Design review of the part built by this model. Coordinates are the model's own, in mm. Round coordinates to 2 decimals unless told otherwise and drop trailing zeros. Loops run counter-clockwise (first coordinate to the right, second up) from the corner with the lowest first, then second, coordinate; pieces in that order, holes last. Notation, with made-up numbers: (-27, -22) -> (21, -22) arc R30 ccw to (21, 16) -> close; hole circle Ø1 at (10.25, -25). An arc over 180 degrees is marked (long way). Answer as CSV lines item,"result". Start each with the question number.
```python
from build123d import *

# Parameters (mm, degrees)
BOSS_EXTRUDE1_DEPTH = 4
SKETCH2_W           = 165.1
SKETCH2_H           = 63.5
CUT_EXTRUDE1_DEPTH  = 349.523826216
CUT_EXTRUDE2_DEPTH  = 10


with BuildPart() as part:
    # Sketch1 → Boss-Extrude1 (new body)
    with BuildSketch(Plane(origin=(0, 0, 0), x_dir=(1, 0, 0), z_dir=(0, 1, 0))):
        Polygon((310, -100), (310, -10), (280.7, -10), (280.7, -6), (310, -6), (310, 0), (0, 0), (0, -6), (29.3, -6), (29.3, -10), (0, -10), (0, -100), (153, -159.225806452), (153, -128.4), (157, -128.4), (157, -159.225806452), align=None)
    extrude(amount=BOSS_EXTRUDE1_DEPTH)

    # Sketch2 → Cut-Extrude1 (cut, through all)
    with BuildSketch(Plane(origin=(0, 4, 0), x_dir=(1, 0, 0), z_dir=(0, 1, 0))):
        with Locations((155, -31.75)):
            Rectangle(SKETCH2_W, SKETCH2_H)
    extrude(amount=-CUT_EXTRUDE1_DEPTH, mode=Mode.SUBTRACT)

    # Sketch4 → Cut-Extrude2 (cut)
    with BuildSketch(Plane(origin=(0, 4, 0), x_dir=(1, 0, 0), z_dir=(0, 1, 0))):
        with BuildLine():
            ThreePointArc((73.3, -97.8), (73.429171307, -98.929171307), (73.810011136, -100))
            Line((73.810011136, -100), (78.3, -100))
            Line((78.3, -100), (78.3, -97.8))
            Line((78.3, -97.8), (73.3, -97.8))
        make_face()
        with BuildLine():
            Line((78.3, -100), (73.810011136, -100))
            ThreePointArc((73.810011136, -100), (79.429171307, -102.670828693), (83.3, -97.8))
            ThreePointArc((83.3, -97.8), (78.3, -92.8), (73.3, -97.8))
            Line((73.3, -97.8), (78.3, -97.8))
            Line((78.3, -97.8), (78.3, -100))
        make_face()
        with BuildLine():
            Line((236.189988864, -100), (231.7, -100))
            Line((231.7, -100), (231.7, -97.8))
            Line((231.7, -97.8), (236.7, -97.8))
            ThreePointArc((236.7, -97.8), (226.829171307, -96.670828693), (236.189988864, -100))
        make_face()
        with BuildLine():
            Line((231.7, -97.8), (231.7, -100))
            Line((231.7, -100), (236.189988864, -100))
            ThreePointArc((236.189988864, -100), (236.570828693, -98.929171307), (236.7, -97.8))
            Line((236.7, -97.8), (231.7, -97.8))
        make_face()
    extrude(amount=-CUT_EXTRUDE2_DEPTH, mode=Mode.SUBTRACT)


solid = part.part
```
Q1. Add section A-A, the plane y = 1.95. Give the boundary of the cut face in (x, z), and give its area (3 significant figures).
Q2. Add section D-D, the plane x = 40. Give the boundary of the cut face in (y, z), and give its area (3 significant figures).
Q3. Add section C-C, the plane x = 108. Give the boundary of the cut face in (y, z), and give its area (3 significant figures).
Q4. To check wall thickness, follow probe 1 along X at (y, z) = (1.3, 97.8); probe 2 along X at (y, z) = (1.7, 40.5); probe 3 along Z at (x, y) = (231.7, 1.7). State the ranges of each line that lie inside material, in increasing order. Write a range as from..to.
Q5. For pin 1 Ø1.2 at (x, y) = (154.5, 3) entering from +Z; pin 2 Ø1.5 at (x, y) = (146.5, 1) entering from +Z; pin 3 Ø8 at (x, z) = (231.7, 97.8) entering from -Y; pin 4 Ø1.2 at (x, y) = (11.5, 1) entering from +Z, all flat-tipped, find the tip position at first contact; note any pin that passes through.
Q6. Add section B-B, the plane x = 231.7. Give the boundary of the cut face in (y, z), and give its area (3 significant figures).
Worked answers:
1,outline,"(0, 0) -> (72.45, 0) -> (72.45, 63.5) -> (237.55, 63.5) -> (237.55, 0) -> (310, 0) -> (310, 6) -> (280.7, 6) -> (280.7, 10) -> (310, 10) -> (310, 100) -> (157, 159.23) -> (157, 128.4) -> (153, 128.4) -> (153, 159.23) -> (0, 100) -> (0, 10) -> (29.3, 10) -> (29.3, 6) -> (0, 6) -> close; hole circle Ø10 at (78.3, 97.8); hole circle Ø10 at (231.7, 97.8)"
1,area,"29,300 mm^2"
2,outline,"(0, 0) -> (4, 0) -> (4, 115.48) -> (0, 115.48) -> close"
2,area,"462 mm^2"
3,outline,"(0, 63.5) -> (4, 63.5) -> (4, 141.81) -> (0, 141.81) -> close"
3,area,"313 mm^2"
4,probe 1,"x = 0..73.3, 83.3..226.7, 236.7..310"
4,probe 2,"x = 0..72.45, 237.55..310"
4,probe 3,"z = 63.5..92.8, 102.8..130.31"
5,pin 1,"stops at z = 128.4"
5,pin 2,"stops at z = 157"
5,pin 3,"passes through"
5,pin 4,"stops at z = 104.68"
6,outline,"(0, 63.5) -> (4, 63.5) -> (4, 92.8) -> (0, 92.8) -> close; (0, 102.8) -> (4, 102.8) -> (4, 130.31) -> (0, 130.31) -> close"
6,area,"227 mm^2"
